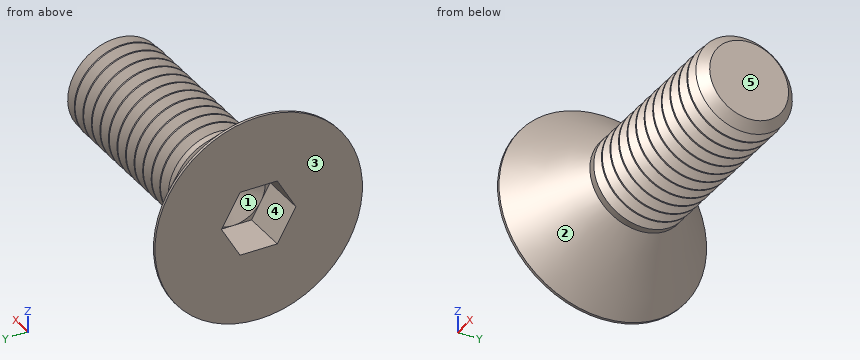
from build123d import *

# Parameters (mm, degrees)
CUT_EXTRUDE1_DEPTH = 2.2098


with BuildPart() as part:
    # Sketch1 → Revolve1 (revolve)
    with BuildSketch(Plane.XY, mode=Mode.PRIVATE) as revolve1_sk:
        Polygon((0, 5.10667), (0, 0), (12.7, 0), (12.7, 1.94056), (12.268263383, 2.372296616), (11.96595815, 1.94056), (11.635152101, 2.413), (11.56269695, 2.413), (11.2318909, 1.94056), (10.901084851, 2.413), (10.8286297, 2.413), (10.49782365, 1.94056), (10.167017601, 2.413), (10.09456245, 2.413), (9.7637564, 1.94056), (9.432950351, 2.413), (9.3604952, 2.413), (9.02968915, 1.94056), (8.698883101, 2.413), (8.62642795, 2.413), (8.2956219, 1.94056), (7.964815851, 2.413), (7.8923607, 2.413), (7.561554651, 1.94056), (7.230748601, 2.413), (7.15829345, 2.413), (6.827487401, 1.94056), (6.496681351, 2.413), (6.4242262, 2.413), (6.093420151, 1.94056), (5.762614101, 2.413), (5.69015895, 2.413), (5.359352901, 1.94056), (5.028546851, 2.413), (4.9560917, 2.413), (4.625285651, 1.94056), (4.294479601, 2.413), (4.22202445, 2.413), (3.891218401, 1.94056), (3.560412352, 2.413), (3.225712867, 2.413), (0.127, 5.10667), align=None)
    revolve(revolve1_sk.sketch.rotate(Axis((0, 0, 0), (1, 0, 0)), 270), axis=Axis((0, 0, 0), (1, 0, 0)))

    # Sketch2 → Cut-Extrude1 (cut)
    with BuildSketch(Plane.ZY):
        Polygon((0, 1.833087105), (-1.5875, 0.916543552), (-1.5875, -0.916543552), (0, -1.833087105), (1.5875, -0.916543552), (1.5875, 0.916543552), align=None)
    extrude(amount=-CUT_EXTRUDE1_DEPTH, mode=Mode.SUBTRACT)

    # Sketch3 → Cut-Revolve1 (revolve, cut)
    with BuildSketch(Plane.XY, mode=Mode.PRIVATE) as cut_revolve1_sk:
        Polygon((2.2098, 1.5875), (2.2098, 0), (3.126343553, 0), align=None)
    revolve(cut_revolve1_sk.sketch.rotate(Axis((2.209775, 0, 0), (1, 0, 0)), 90), axis=Axis((2.209775, 0, 0), (1, 0, 0)), mode=Mode.SUBTRACT)


solid = part.part
Geometry check sheet. Reference: the model listing, model coordinates, mm. Face numbers are marked on the shaded views. A direction names the side the tool comes from. Coordinates: 2 decimals unless noted, no trailing zeros. Use one line per item in the form item = value. Start each with the question number.
Item 1: Mould release check, pull along Z, two halves, no side actions. Record for the marked faces 1, 2 and 3: +Z half, -Z half, draft (parallel to the pull), parting line (faces both ways), or undercut.
Item 2: Gauge pin test, flat ends, axial feed: pin 1 (1.5 mm diameter, centred on x = 8, y = -3.5, fed in from -Z); pin 2 (1.5 mm diameter, centred on x = 1, y = 0.5, fed in from -Z); pin 3 (0.6 mm diameter, centred on y = 0.5, z = 1, fed in from -X); pin 4 (0.5 mm diameter, centred on y = -1.5, z = 0, fed in from -X). Record the tip position at first contact, or that the pin passes through.
Item 3: Tool access check on the marked faces 4 and 5. Record the directions out of +Z, -Z, +X, -X, +Y, -Y that give a thin tool (end or side, any length) a straight path to the whole face; none if there is none.
Item 4: Thickness scan on probe 1 along Y at (x, z) = (9, 0.75); probe 2 along Y at (x, z) = (2, -2.5); probe 3 along Z at (x, y) = (2, 0). Record the ranges inside material, lowest first.
Computed:
q1.face_1 = undercut
q1.face_2 = parting line
q1.face_3 = draft
q2.pin_1 = through
q2.pin_2 = -4.98
q2.pin_3 = 2.31
q2.pin_4 = 2.21
q3.face_4 = -X
q3.face_5 = +Z, -Z, +X, +Y, -Y
q4.probe_1 = -1.84 to 1.84
q4.probe_2 = -2.42 to 2.42
q4.probe_3 = -3.48 to -1.59, 1.59 to 3.48
